Verification items for the finished model (mm, model axes). A direction names the side the tool comes from. Round coordinates to 2 decimals unless told otherwise and drop trailing zeros. Write each loop counter-clockwise with the first axis right and the second up, starting at its lowest first coordinate (ties: lowest second). Pieces come first, ordered by that corner, then holes. Notation, with made-up numbers: (46.25, -25.75) - (61.25, -25.75) arc R21 ccw to (61.25, 6.25) - close; hole circle Ø3 at (-6, 70.25). An arc over 180 degrees is marked (long way). Answer as a JSON object with one key per item and string values. Group by question number.
1) Section check A-A (z = 0). State how many separate pieces and enclosed holes the cut face has, then the cut area to 3 significant figures.
2) Thickness scan on line 1 (Y direction, x = -6.1, z = 0) (3 decimals); line 2 (X direction, y = 3.25, z = 0.5); line 3 (X direction, y = 2.25, z = -2). Record the ranges inside material, lowest first.
3) Set-up check for faces 1 (the cylindrical face through (-2.651, 6.098, 1.198)), 2 (the flat face through (-5.6, -3.6, 1.4)), 3 (the flat face through (-3.1, 6.3, 1.4)), 4 (the cylindrical face through (2.53, -0.11, -0.33)): record each of +Z, -Z, +X, -X, +Y, -Y from which the full face is reachable in a straight line by a thin tool's end or side.
4) Mould release check, pull along Z, two halves, no side actions. Record for faces 5 (the flat face through (2, -8, -2)), 6 (the cylindrical face through (7.684, -0.112, -1.009)), 7 (the flat face through (-3.1, -3.6, 1.4)), 8 (the flat face through (-4, 5, -3.1)): +Z half, -Z half, draft (parallel to the pull), parting line (faces both ways), or undercut.
5) Section check B-B (x = 0). Enter the section's corners in (y, z).
6) Section check C-C (y = -2.75). Enter the section's corners in (x, z).
7) Go/stop test with flat-tipped pins: pin 1 Ø1.5 at (x, y) = (-4, -2) entering from -Z; pin 2 Ø4 at (x, y) = (-3, -2.5) entering from -Z; pin 3 Ø4.5 at (x, z) = (0, 0) entering from -Y; pin 4 Ø2 at (x, z) = (-4.5, -1) entering from +Y. Record where each tip stops, or that it passes through.
8) Section check D-D (x = -5). Enter the section's corners in (y, z).
```python
from build123d import *

# Parameters (mm, degrees)
BOSS_EXTRUDE2_DEPTH      = 8
BOSS_EXTRUDE2_DEPTH_BACK = 8
SKETCH1_R                = 7.75
SKETCH1_R_2              = 2.55
SKETCH2_R                = 1.625
CUT_EXTRUDE1_DEPTH       = 20.5
CUT_EXTRUDE2_START       = -3.1
SKETCH4_W                = 6.2
SKETCH4_H                = 6.1
CUT_EXTRUDE2_DEPTH       = 2.5


with BuildPart() as part:
    # Sketch1 → Boss-Extrude2 (new, two sides: drawn at the far end of the back side and taken through both)
    with BuildSketch(Plane(origin=(0, 0, 0), x_dir=(1, 0, 0), z_dir=(0, 1, 0)).offset(-BOSS_EXTRUDE2_DEPTH_BACK)):
        with Locations(Location((0, 0, 0), (0, 0, 270))):
            Circle(SKETCH1_R)
        with Locations(Location((0, 0, 0), (0, 0, 270))):
            Circle(SKETCH1_R_2, mode=Mode.SUBTRACT)
    extrude(amount=BOSS_EXTRUDE2_DEPTH + BOSS_EXTRUDE2_DEPTH_BACK)

    # Sketch2 → Cut-Extrude1 (cut)
    with BuildSketch(Plane(origin=(0, 0, 0), x_dir=(0, 0, -1), z_dir=(1, 0, 0))):
        with Locations((0, 5)):
            Circle(SKETCH2_R)
        with Locations((0, -5)):
            Circle(SKETCH2_R)
    extrude(amount=-CUT_EXTRUDE1_DEPTH, mode=Mode.SUBTRACT)

    # Sketch4 → Cut-Extrude2 (cut)
    with BuildSketch(Plane(origin=(0, 0, 0), x_dir=(0, 0, -1), z_dir=(1, 0, 0)).offset(CUT_EXTRUDE2_START)):
        with Locations((0, 4.95)):
            Rectangle(SKETCH4_W, SKETCH4_H)
        with Locations((0, -4.95)):
            Rectangle(SKETCH4_W, SKETCH4_H)
    extrude(amount=-CUT_EXTRUDE2_DEPTH, mode=Mode.SUBTRACT)


solid = part.part
```
Returned:
{
 "1": {"separate pieces": "6", "enclosed holes": "0", "area": "118 mm2"},
 "2": {"line 1": "-8 to -6.625, -3.375 to 3.375, 6.625 to 8", "line 2": "-7.73 to -5.6, -3.1 to -2.5, 2.5 to 7.73", "line 3": "-7.49 to -5.6, -3.1 to -1.58, 1.58 to 7.49"},
 "3": {"face 1": "-X", "face 2": "-Y", "face 3": "+Y", "face 4": "+Y, -Y"},
 "4": {"face 5": "draft", "face 6": "parting line", "face 7": "undercut", "face 8": "undercut"},
 "5": {"outline": "(-8, -7.75) - (8, -7.75) - (8, -2.55) - (-8, -2.55) - close; (-8, 2.55) - (8, 2.55) - (8, 7.75) - (-8, 7.75) - close"},
 "6": {"outline": "circle Ø15.5 at (0, 0); hole (-5.6, -3.1) - (-3.1, -3.1) - (-3.1, 3.1) - (-5.6, 3.1) - close; hole circle Ø5.1 at (0, 0)"},
 "7": {"pin 1": "z = -7.04", "pin 2": "z = -7.69", "pin 3": "through", "pin 4": "y = 1.9"},
 "8": {"outline": "(-8, -5.92) - (8, -5.92) - (8, -3.1) - (1.9, -3.1) - (1.9, 3.1) - (8, 3.1) - (8, 5.92) - (-8, 5.92) - (-8, 3.1) - (-1.9, 3.1) - (-1.9, -3.1) - (-8, -3.1) - close"}
}
